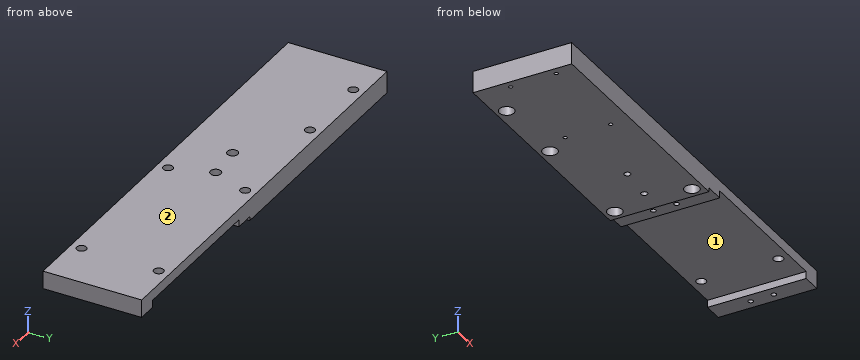
Autodesk Inventor part; units mm, degrees
ref_plane "YZ Plane" through (0, 0, 0) normal (1, 0, 0) x (0, 1, 0)
ref_plane "XZ Plane" through (0, 0, 0) normal (0, 1, 0) x (-1, 0, 0)
ref_plane "XY Plane" through (0, 0, 0) normal (0, 0, 1) x (1, 0, 0)
sketch "Sketch1" plane through (0, 0, 0) normal (0, 0, 1) x (1, 0, 0)
  line L0 (-192.5, 32.5) -> (192.5, 32.5)
  line L1 (192.5, 32.5) -> (192.5, -32.5)
  line L2 (192.5, -32.5) -> (-192.5, -32.5)
  line L3 (-192.5, -32.5) -> (-192.5, 32.5)
  point P0 (0, 0)
  dimension "d0" = 385
  dimension "d1" = 192.5
  dimension "d2" = 65
  dimension "d3" = 32.5
extrude "Extrusion1" add sketch "Sketch1" along normal blind 7
sketch "Sketch2" plane through (0, 0, 0) normal (0, 0, -1) x (-1, 0, 0)
  line L0 (192.5, 32.5) -> (-192.5, 32.5)
  line L1 (-192.5, 32.5) -> (-192.5, -32.5)
  line L2 (-192.5, -32.5) -> (192.5, -32.5)
  line L3 (17.417, 16.6256) -> (17.417, -16.6484)
  line L4 (-192.5, 16.6256) -> (-192.5, -16.6484)
  line L5 (17.417, 32.5) -> (17.417, -32.5)
  line L6 (4.717, 16.6256) -> (4.717, -16.6484)
  line L7 (-171.164, 18.034) -> (-179.8, 18.034)
  line L8 (-179.8, 16.6256) -> (-179.8, -16.6484)
  line L9 (-179.8, 32.5) -> (-179.8, -32.5)
  line L10 (4.717, 32.5) -> (4.717, -32.5)
  point P0 (0, 0)
extrude "Extrusion2" add sketch "Sketch2" along normal blind 4.7408 contours L5 L3 L2 L10 L6 L0 | L9 L8 L2 L1 L0
sketch "Sketch3" plane through (0, 0, 0) normal (0, 0, -1) x (-1, 0, 0)
  line L0 (17.417, 32.5) -> (17.417, -32.5)
  line L1 (17.417, -32.5) -> (192.5, -32.5)
  line L2 (63.2414, 16.4628) -> (60.0979, -19.4679)
  line L3 (17.417, 32.5) -> (67.417, 32.5)
  line L4 (67.417, 32.5) -> (67.417, -32.5)
  line L5 (67.417, -32.5) -> (17.417, -32.5)
  line L6 (17.417, -32.5) -> (17.417, 32.5)
  line L7 (76.6696, -19.4) -> (76.6696, 30.6)
  line L8 (17.417, 32.5) -> (76.6696, 32.5)
  line L9 (76.6696, -32.5) -> (17.417, -32.5)
  line L10 (17.417, -32.5) -> (17.417, 32.5)
  circle A0 centre (83.6696, -4.5) radius 1.5
  circle A1 centre (83.6696, 10.5) radius 2
  line L11 (87.4689, -18.5) -> (87.4689, -24.5)
  line L12 (88.6696, -24.5) -> (87.4689, -24.5)
  line L13 (88.6696, 15.5) -> (88.6696, -24.5)
  line L14 (78.6696, 15.5) -> (88.6696, 15.5)
  line L15 (78.6696, -15.5) -> (78.6696, 15.5)
  line L16 (78.6696, -15.5) -> (84.4689, -15.5)
  arc A2 (87.4689, -18.5) -> (84.4689, -15.5) centre (84.4689, -18.5) ccw
  line L17 (67.417, 32.5) -> (78.6696, 32.5)
  line L18 (78.6696, 32.5) -> (78.6696, -32.5)
  line L19 (78.6696, -32.5) -> (67.417, -32.5)
  line L20 (67.417, -32.5) -> (67.417, 32.5)
  point P0 (0, 0)
  dimension "d8" = 50
  dimension "d11" = 0
extrude "Extrusion3" add sketch "Sketch3" along normal blind 7.3198 contours L3 L4 L1 L0 | L8 L17 L18 L15 L1 L4
sketch "Sketch6" plane through (-192.5, -32.5, 7) normal (-1, 0, 0) x (0, 0, 1)
  line L0 (-23, 0) -> (-23, 65)
  circle A0 centre (-28, 23.1) radius 1.2295
  circle A1 centre (-28, 53.1) radius 1.2295
  point P0 (-7, 32.5)
hole "Hole1" at (-192.5, -9.4, -21) at (-192.5, 20.6, -21) direction (1, 0, 0) diameter 3 end through all counterbore diameter 5.75 counterbore depth 3
sketch "Sketch8" plane through (0, 0, 7) normal (0, 0, 1) x (1, 0, 0)
  circle A0 centre (-57.2416, -1.1152) radius 2.0828
  circle A1 centre (-33.7068, 0.9439) radius 2.0828
  point P0 (0, 0)
hole "Hole3" at (-33.7068, 0.9439, 7) at (-57.2416, -1.1152, 7) direction (0, 0, -1) diameter 4.1656 end through all counterbore diameter 6.985 counterbore depth 5
sketch "Sketch9" plane through (0, 0, -4.7408) normal (0, 0, -1) x (-1, 0, 0)
  circle A0 centre (11.067, -7.6314) radius 2.1844
  circle A1 centre (11.067, 7.6086) radius 2.1844
  circle A2 centre (-186.15, -7.6314) radius 2.1844
  circle A3 centre (-186.15, 7.6086) radius 2.1844
  point P0 (0, 0)
hole "Hole4" at (-11.067, -7.6314, -4.7408) at (-11.067, 7.6086, -4.7408) at (186.15, -7.6314, -4.7408) at (186.15, 7.6086, -4.7408) direction (0, 0, 1) diameter 3.302 depth 8 tip angle 118
sketch "Sketch10" plane through (0, 0, 0) normal (0, 0, -1) x (-1, 0, 0)
  line L0 (192.5, 32.5) -> (78.6696, 32.5)
  line L1 (178.6696, 15.5) -> (178.6696, -24.5)
  line L2 (178.6696, 32.5) -> (192.5, 32.5)
  line L3 (192.5, 32.5) -> (192.5, -32.5)
  line L4 (192.5, -32.5) -> (178.6696, -32.5)
  line L5 (178.6696, -32.5) -> (178.6696, 32.5)
  point P0 (0, 0)
extrude "Extrusion6" cut sketch "Sketch10" against normal blind 10
sketch "Sketch11" plane through (0, 0, 0) normal (0, 0, -1) x (-1, 0, 0)
  line L0 (178.6696, -32.5) -> (178.6696, 32.5)
  line L1 (178.6696, 32.5) -> (78.6696, 32.5)
  line L2 (78.6696, 32.5) -> (78.6696, -32.5)
  line L3 (78.6696, -32.5) -> (178.6696, -32.5)
  point P0 (0, 0)
extrude "Extrusion7" add sketch "Sketch11" along normal blind 7.3198
sketch "Sketch12" plane through (0, 0, -7.3198) normal (0, 0, -1) x (-1, 0, 0)
  circle A0 centre (173.6696, 10.5) radius 2
  circle A1 centre (173.6696, -19.5) radius 2
  line L0 (78.6696, 15.5) -> (178.6696, 15.5)
  line L1 (178.6696, 15.5) -> (178.6696, -24.5)
  line L2 (178.6696, -24.5) -> (78.6696, -24.5)
  line L3 (78.6696, -24.5) -> (78.6696, 15.5)
  circle A2 centre (109.6696, -19.5) radius 2.0298
  circle A3 centre (109.6696, 10.5) radius 2
  point P0 (0, 0)
  dimension "d126" = 64
  dimension "d127" = 30
  dimension "d128" = 64
hole "Hole5" at (-173.6696, 10.5, -7.3198) at (-173.6696, -19.5, -7.3198) direction (0, 0, 1) diameter 2.459 depth 8.8 tip angle 118
sketch "Sketch13" plane through (0, 0, -7.3198) normal (0, 0, -1) x (-1, 0, 0)
  line L0 (171.6696, -6) -> (175.6696, -6)
  arc A0 (175.6696, -6) -> (175.6696, -3) centre (175.6696, -4.5) ccw
  line L1 (175.6696, -3) -> (171.6696, -3)
  arc A1 (171.6696, -3) -> (171.6696, -6) centre (171.6696, -4.5) ccw
  circle A2 centre (83.6696, -4.5) radius 1.5
  circle A3 centre (173.6696, 10.5) radius 2
  circle A4 centre (173.6696, -19.5) radius 2
  circle A5 centre (83.6696, 10.5) radius 2
  circle A6 centre (83.6696, -19.5) radius 2
  line L2 (78.6696, 15.5) -> (178.6696, 15.5)
  line L3 (178.6696, 15.5) -> (178.6696, -24.5)
  line L4 (178.6696, -24.5) -> (78.6696, -24.5)
  line L5 (78.6696, -24.5) -> (78.6696, 15.5)
  point P0 (0, 0)
  point P1 (173.6696, -4.5)
hole "Hole6" [suppressed]
sketch "Sketch14" plane through (0, 0, -7.3198) normal (0, 0, -1) x (-1, 0, 0)
  circle A0 centre (126.3, 25.4) radius 3.175
  circle A1 centre (151.7, 25.4) radius 3.175
  point P0 (0, 0)
  point P1 (100.9, 25.4)
  dimension "d63" = 50.8
hole "Hole7" at (-151.7, 25.4, -7.3198) at (-100.9, 25.4, -7.3198) direction (0, 0, 1) diameter 6.35 end through all counterbore diameter 9.652 counterbore depth 7
sketch "Sketch15" plane through (0, 0, -7.3198) normal (0, 0, -1) x (-1, 0, 0)
  line L0 (17.417, 32.5) -> (78.6696, 32.5)
  circle A0 centre (100.9, 25.4) radius 4.826
  point P0 (0, 0)
  point P1 (24.7, 25.4)
  point P2 (24.7, -25.4)
  dimension "d71" = 7.1
  dimension "d72" = 76.2
  dimension "d73" = 76.2
  dimension "d74" = 50.8
hole "Hole8" at (-24.7, 25.4, -7.3198) at (-24.7, -25.4, -7.3198) direction (0, 0, 1) diameter 6.35 end through all counterbore diameter 9.652 counterbore depth 7
sketch "Sketch17" plane through (0, 0, 0) normal (0, 0, -1) x (-1, 0, 0)
  line L0 (-179.8, -32.5) -> (4.717, -32.5)
  line L1 (4.717, 32.5) -> (-179.8, 32.5)
  line L2 (-109.583, 16.6256) -> (-109.583, -16.6484)
  line L3 (-96.883, 16.6256) -> (-96.883, -16.6484)
  line L4 (-96.883, 32.5) -> (-109.583, 32.5)
  line L5 (-109.583, 32.5) -> (-109.583, -32.5)
  line L6 (-109.583, -32.5) -> (-96.883, -32.5)
  line L7 (-96.883, -32.5) -> (-96.883, 32.5)
  point P0 (0, 0)
extrude "Extrusion8" add sketch "Sketch17" along normal blind 4.7408
sketch "Sketch18" plane through (0, 0, -4.7408) normal (0, 0, -1) x (-1, 0, 0)
  circle A0 centre (-103.233, -7.6314) radius 2.1844
  circle A1 centre (-103.233, 7.6086) radius 2.1844
  point P0 (0, 0)
hole "Hole10" at (103.233, -7.6314, -4.7408) at (103.233, 7.6086, -4.7408) direction (0, 0, 1) diameter 3.302 depth 8 tip angle 118
sketch "Sketch19" plane through (0, 0, -4.7408) normal (0, 0, -1) x (-1, 0, 0)
  line L0 (-192.5, -32.5) -> (-192.5, 32.5)
  line L1 (-179.8, -32.5) -> (-109.583, -32.5)
  line L2 (-109.583, 32.5) -> (-179.8, 32.5)
  line L3 (-109.583, 32.5) -> (-192.5, 32.5)
  line L4 (-192.5, 32.5) -> (-192.5, -32.5)
  line L5 (-192.5, -32.5) -> (-109.583, -32.5)
  line L6 (-109.583, -32.5) -> (-109.583, 32.5)
  point P0 (0, 0)
extrude "Extrusion9" cut sketch "Sketch19" against normal blind 25
sketch "Sketch20" plane through (0, 0, 0) normal (0, 0, -1) x (-1, 0, 0)
  circle A0 centre (24.7, -25.4) radius 4.826
  circle A1 centre (24.7, 25.4) radius 4.826
  point P0 (0, 0)
  point P1 (-76.9, -25.4)
  point P2 (-76.9, 25.4)
  dimension "d103" = 101.6
  dimension "d104" = 101.6
hole "Hole11" at (76.9, -25.4, 0) at (76.9, 25.4, 0) direction (0, 0, 1) diameter 6.35 end through all
hole "Hole12" at (-109.6696, 10.5, -7.3198) direction (0, 0, 1) diameter 2.459 depth 8.8 tip angle 118
hole "Hole13" at (-109.6696, -19.5, -7.3198) direction (0, 0, 1) diameter 2.459 depth 8.8 tip angle 118
properties part number "OBIS laser subassy shortened baseplate"
Verification items for the finished model (mm, model axes). Face numbers are marked on the shaded views. A direction names the side the tool comes from. Coordinates: 2 decimals unless noted, no trailing zeros. Loops run counter-clockwise (first coordinate to the right, second up) from the corner with the lowest first, then second, coordinate; pieces in that order, holes last. Notation, with made-up numbers: (-0.75, 9) - (27.25, 9) arc R21 cw to (27.25, 41) - close; hole circle Ø2 at (60, -23.5). An arc over 180 degrees is marked (long way). Return JSON: item names as keys, results as strings.
1. Section check A-A, the plane x = 76.9. Record the boundary of the cut face in (y, z) (3 decimals).
Established:
{"outline": "(-32.5, 0) - (-28.575, 0) - (-28.575, 7) - (-32.5, 7) - close; (-22.225, 0) - (22.225, 0) - (22.225, 7) - (-22.225, 7) - close; (28.575, 0) - (32.5, 0) - (32.5, 7) - (28.575, 7) - close"}
2. Tool access check on the marked faces 1 and 2. Record the directions out of +Z, -Z, +X, -X, +Y, -Y that give a thin tool (end or side, any length) a straight path to the whole face; none if there is none.
Established:
{"face 1": "-Z, +Y, -Y", "face 2": "+Z, +X, -X, +Y, -Y"}
3. Go/stop test with flat-tipped pins: pin 1 (15.5 mm diameter, centred on x = -24.7, y = -25.4, fed in from +Z); pin 2 (10 mm diameter, centred on x = 104, y = -7.5, fed in from -Z). Record where each tip stops, or that it passes through.
Established:
{"pin 1": "stops at z = 7", "pin 2": "stops at z = -4.74"}
4. Thickness scan on L1, parallel to X at y = -19.5, z = -4.25; L2, parallel to X at y = -25.4, z = 3 (3 decimals); L3, parallel to Y at x = 76.9, z = 2.5 (3 decimals). Record the ranges inside material, lowest first.
Established:
{"L1": "x = -178.67 to -174.9, -172.44 to -110.9, -108.44 to -4.72, 96.88 to 109.58", "L2": "x = -178.67 to -27.875, -21.525 to 73.725, 80.075 to 109.583", "L3": "y = -32.5 to -28.575, -22.225 to 22.225, 28.575 to 32.5"}
5. Section check D-D, the plane z = -2.5. Count the separate pieces of the cut face and the enclosed holes in it, then the cut area to 3 significant figures.
Established:
{"separate pieces": "2", "enclosed holes": "14", "area": "11,800 mm2"}
6. Section check B-B, the plane y = -25.4. Record the boundary of the cut face in (x, z) (3 decimals).
Established:
{"outline": "(-178.67, -7.32) - (-29.526, -7.32) - (-29.526, -0.32) - (-27.875, -0.32) - (-27.875, 7) - (-178.67, 7) - close; (-21.525, -0.32) - (-19.874, -0.32) - (-19.874, -7.32) - (-17.417, -7.32) - (-17.417, -4.741) - (-4.717, -4.741) - (-4.717, 0) - (73.725, 0) - (73.725, 7) - (-21.525, 7) - close; (80.075, 0) - (96.883, 0) - (96.883, -4.741) - (109.583, -4.741) - (109.583, 7) - (80.075, 7) - close"}
7. Section check C-C, the plane x = -100.9. Record the boundary of the cut face in (y, z) (3 decimals).
Established:
{"outline": "(-32.5, -7.32) - (20.574, -7.32) - (20.574, -0.32) - (22.225, -0.32) - (22.225, 7) - (-32.5, 7) - close; (28.575, -0.32) - (30.226, -0.32) - (30.226, -7.32) - (32.5, -7.32) - (32.5, 7) - (28.575, 7) - close"}
